Part model, mm, in its own coordinate system. Round coordinates to 2 decimals unless told otherwise and drop trailing zeros. Loops run counter-clockwise (first coordinate to the right, second up) from the corner with the lowest first, then second, coordinate; pieces in that order, holes last.
from build123d import *

# Parameters (mm, degrees)
RESSALTO_EXTRUS_O1_DEPTH = 12.26


with BuildPart() as part:
    # Esboço1 → Ressalto-extrusão1 (new body)
    with BuildSketch(Plane(origin=(0, 0, 0), x_dir=(1, 0, 0), z_dir=(0, 1, 0))):
        with BuildLine():
            ThreePointArc((27.862912529, -17.68214086), (32.657820254, 4.739913109), (21.6864187, 24.873665672))
            Line((21.6864187, 24.873665672), (24.193905015, 31.85365959))
            ThreePointArc((24.193905015, 31.85365959), (14.449004884, 37.299154508), (3.578740021, 39.839594489))
            Line((3.578740021, 39.839594489), (2.684054455, 29.879689618))
            ThreePointArc((2.684054455, 29.879689618), (29.627442083, 4.713244699), (11.823645173, -27.571750304))
            Line((11.823645173, -27.571750304), (12.993920826, -30.334106573))
            Line((12.993920826, -30.334106573), (20.795690346, -48.749654144))
            ThreePointArc((20.795690346, -48.749654144), (24.072464244, -50.130779062), (25.453589161, -46.854005164))
            Line((25.453589161, -46.854005164), (25.198608413, -46.380200094))
            Line((25.198608413, -46.380200094), (15.823293166, -28.958995034))
            ThreePointArc((15.823293166, -28.958995034), (21.396881696, -25.123165678), (26.071005915, -20.231229586))
            ThreePointArc((26.071005915, -20.231229586), (26.997061933, -18.977846216), (27.862912529, -17.68214086))
        make_face()
    extrude(amount=RESSALTO_EXTRUS_O1_DEPTH)


solid = part.part
1) Slice it at D-D, the plane x = 23. Give the cut face in (y, z).
Values:
outline: (0, -32.73) - (12.26, -32.73) - (12.26, -28.53) - (0, -28.53) - close; (0, -23.66) - (12.26, -23.66) - (12.26, -19.26) - (0, -19.26) - close; (0, 19.26) - (12.26, 19.26) - (12.26, 23.66) - (0, 23.66) - close; (0, 42.29) - (12.26, 42.29) - (12.26, 50.31) - (0, 50.31) - close
2) Slice it at A-A, the plane x = 19.5. Give the cut face in (y, z).
Values:
outline: (0, -34.92) - (12.26, -34.92) - (12.26, -22.8) - (0, -22.8) - close; (0, 22.8) - (12.26, 22.8) - (12.26, 26.62) - (0, 26.62) - close; (0, 35.79) - (12.26, 35.79) - (12.26, 45.69) - (0, 45.69) - close
3) Slice it at B-B, the plane x = 14. Give the cut face in (y, z).
Values:
outline: (0, -37.47) - (12.26, -37.47) - (12.26, -26.53) - (0, -26.53) - close; (0, 26.53) - (12.26, 26.53) - (12.26, 32.71) - (0, 32.71) - close
4) Slice it at C-C, the plane y = 1.75. Give the cut face in (x, z), then the cut area to 3 significant figures.
Values:
outline: (2.68, -29.88) - (3.58, -39.84) arc R40 ccw to (24.19, -31.85) - (21.69, -24.87) arc R33 ccw to (15.82, 28.96) - (25.45, 46.85) arc R2.51 ccw to (20.8, 48.75) - (11.82, 27.57) arc R30 cw to start
area: 493 mm2
5) Wall check: line 1 along Z through (x, y) = (20, 3.5); line 2 along Z through (x, y) = (16, 11.75); line 3 along Z through (x, y) = (15, 3). Give the ranges that are in metal, low to high.
Values:
line 1: z = -34.64 to -22.36, 22.36 to 26.25, 36.72 to 46.87
line 2: z = -36.66 to -25.38, 25.38 to 28.86, 29.29 to 37.43
line 3: z = -37.08 to -25.98, 25.98 to 35.07
6) Drop flat-ended pins along their axis: pin 1 Ø6 at (y, z) = (9.5, -3.5) entering from +X; pin 2 Ø3 at (y, z) = (5.5, -14.5) entering from +X; pin 3 Ø1.5 at (y, z) = (2.5, 5.5) entering from +X. Give the stop position or say it passes through.
Values:
pin 1: stops at x = 33
pin 2: stops at x = 30.33
pin 3: stops at x = 32.66
7) Mould opens along Z. For faces 1 (the face through (22.92, 6.04, -28.31)), 2 (the face through (3.138, 6.044, -34.929)), 3 (the face through (28, 12.26, -12)) say: released by +Z, released by -Z, zero draft, split by the parting line, or undercut.
Values:
face 1: undercut
face 2: released by -Z
face 3: zero draft
